Verification items for the finished model (mm, model axes). A direction names the side the tool comes from. Give positions to 0.01 mm unless a question says otherwise; leave off trailing zeros. Write each loop counter-clockwise with the first axis right and the second up, starting at its lowest first coordinate (ties: lowest second). Pieces come first, ordered by that corner, then holes. Notation, with made-up numbers: (38.25, 6) - (47.25, 6) arc R19 ccw to (47.25, 15) - close; hole circle Ø9 at (1.5, 86.25). An arc over 180 degrees is marked (long way). Answer as a JSON object with one key per item and string values. Group by question number.
Item 1: Sectioned sample at D-D, the plane x = 10. Record the boundary of the cut face in (y, z), and give its area (3 significant figures).
Item 2: Sectioned sample at C-C, the plane z = 5. Count the separate pieces of the cut face and the enclosed holes in it, and give its area (3 significant figures).
Item 3: Sectioned sample at A-A, the plane y = 0. Record the boundary of the cut face in (x, z).
Item 4: Scan lines: line 1 along X through (y, z) = (-14.5, 3.25); line 2 along X through (y, z) = (-5, 9.5); line 3 along Y through (x, z) = (12.5, 5.75). Record each from-to range of solid material in increasing order. Write a range as [from, to].
Item 5: Tool access check on faces 4 (the face through (-1.172, -8.923, 1.972)), 5 (the face through (10.373, 14.094, 5.754)), 6 (the face through (7, 10, 4)), 7 (the face through (0, -15, 10)). Record the directions out of +Z, -Z, +X, -X, +Y, -Y that give a thin tool (end or side, any length) a straight path to the whole face; none if there is none.
Item 6: Draft check along Y on faces 1 (the face through (-7.79, -9.84, 5.96)), 2 (the face through (9, 12, 10)), 3 (the face through (-7, 7, 14)). Enter one of: +Y half, -Y half, draft (parallel to the pull), parting line (faces both ways), or undercut.
Item 7: Go/stop test with flat-tipped pins: pin 1 (3.5 mm diameter, centred on x = 9.4, y = -12.94, fed in from +Z); pin 2 (2 mm diameter, centred on y = 2, z = 2, fed in from -X); pin 3 (5 mm diameter, centred on y = -13.5, z = 5, fed in from +X); pin 4 (6 mm diameter, centred on y = 9, z = 8, fed in from +X). Record where each tip stops, or that it passes through.
Item 8: Sectioned sample at B-B, the plane x = 0. Record the boundary of the cut face in (y, z), and give its area (3 significant figures).
Autodesk Fusion 360 part; units mm, degrees
sketch "Sketch1" plane through (0, 0, 0) normal (0, 0, 1) x (1, 0, 0)
  circle A0 centre (0, 0) radius 9
  circle A1 centre (0, 0) radius 16 construction
  line L0 (0, 0) -> (0, 16) construction
  circle A2 centre (0, 16) radius 3.5
  circle A3 centre (-15.2169, 4.9443) radius 3.5
  circle A4 centre (-9.4046, -12.9443) radius 3.5
  circle A5 centre (9.4046, -12.9443) radius 3.5
  circle A6 centre (15.2169, 4.9443) radius 3.5
  circle A7 centre (0, 0) radius 15
  circle A8 centre (0, 0) radius 21
  circle A9 centre (0, 0) radius 12 construction
  line L1 (0, 0) -> (-8.8168, 12.1353) construction
  circle A10 centre (-7.0534, 9.7082) radius 2
  circle A11 centre (-7.0534, 9.7082) radius 2.25 construction
  circle A12 centre (-11.4127, -3.7082) radius 2
  circle A13 centre (0, -12) radius 2
  circle A14 centre (11.4127, -3.7082) radius 2
  circle A15 centre (7.0534, 9.7082) radius 2
  line L2 (0, 0) -> (-15.2169, 4.9443) construction
  circle A16 centre (0, 16) radius 2.25
  circle A17 centre (-15.2169, 4.9443) radius 2.25
  circle A18 centre (-9.4046, -12.9443) radius 2.25
  circle A19 centre (9.4046, -12.9443) radius 2.25
  circle A20 centre (15.2169, 4.9443) radius 2.25
  circle A21 centre (0, 0) radius 8.5
  dimension "d1" = 18
  dimension "d3" = 7
  dimension "d5" = 360
  dimension "d6" = 30
  dimension "d7" = 42
  dimension "d8" = 4
  dimension "d9" = 4.5
  dimension "d10" = 24
  dimension "d12" = 360
  dimension "d13" = 36
  dimension "d14" = 72
  dimension "d17" = 4.5
  dimension "d19" = 360
  dimension "d26" = 17
  dimension "d31" = 32
extrude "Extrude1" add sketch "Sketch1" along normal blind 6 contours A2 A3 A4 A5 A6 A7 | A8
extrude "Extrude6" add sketch "Sketch1" along normal blind 14 contours A2 A3 A4 A5 A6 A7
extrude "Extrude7" add sketch "Sketch1" along normal blind 1 contours A2 A7 A16 | A2 A7 A16 | A3 A7 A17 | A3 A7 A17 | A6 A7 A20 | A6 A7 A20 | A4 A7 A18 | A4 A7 A18 | A5 A7 A19 | A5 A7 A19
extrude "Extrude4" add sketch "Sketch1" along normal blind 14 contours A0
extrude "Extrude5" cut sketch "Sketch1" along normal blind 4 contours A0
sketch "Sketch2" plane through (0, 0, 6) normal (0, 0, 1) x (-1, 0, 0)
  circle A0 centre (0, 0) radius 21
  arc A1 (-12.9338, -7.5971) -> (-3.2285, -14.6484) centre (0, 0) ccw
  arc A2 (-14.9292, -1.4561) -> (-12.9338, -7.5971) centre (-15.2169, -4.9443) ccw
  arc A3 (-11.2221, 9.9532) -> (-14.9292, -1.4561) centre (0, 0) ccw
  arc A4 (-5.9982, 13.7485) -> (-11.2221, 9.9532) centre (-9.4046, 12.9443) ccw
  arc A5 (5.9982, 13.7485) -> (-5.9982, 13.7485) centre (0, 0) ccw
  arc A6 (11.2221, 9.9532) -> (5.9982, 13.7485) centre (9.4046, 12.9443) ccw
  arc A7 (14.9292, -1.4561) -> (11.2221, 9.9532) centre (0, 0) ccw
  arc A8 (12.9338, -7.5971) -> (14.9292, -1.4561) centre (15.2169, -4.9443) ccw
  arc A9 (3.2285, -14.6484) -> (12.9338, -7.5971) centre (0, 0) ccw
  arc A10 (-3.2285, -14.6484) -> (3.2285, -14.6484) centre (0, -16) ccw
  circle A11 centre (0, 0) radius 17.5
  dimension "d36" = 35
extrude "Extrude8" cut sketch "Sketch2" against normal blind 0.5
sketch "Sketch3" plane through (0, 0, 0) normal (0, 0, -1) x (1, 0, 0)
  circle A0 centre (0, 0) radius 9
  circle A1 centre (-9.4046, 12.9443) radius 2.25
  circle A2 centre (-15.2169, -4.9443) radius 2.25
  circle A3 centre (9.4046, 12.9443) radius 2.25
  circle A4 centre (0, -16) radius 2.25
  circle A5 centre (15.2169, -4.9443) radius 2.25
  circle A6 centre (-7.0534, -9.7082) radius 2
  circle A7 centre (11.4127, 3.7082) radius 2
  circle A8 centre (0, 12) radius 2
  circle A9 centre (7.0534, -9.7082) radius 2
  circle A10 centre (-11.4127, 3.7082) radius 2
  circle A11 centre (0, 0) radius 21
extrude "Extrude9" add sketch "Sketch3" against normal blind 4 contours A6 | A7 | A8 | A9 | A10
equation "d10 = ( d6 - d1 ) / 2 + d1"
equation "d13 = d14 / 2"
Geometry check:
{
 "1": {"outline": "(-18.47, 0) - (-15.11, 0) - (-15.11, 1) - (-16.39, 1) - (-16.39, 5.5) - (-18.47, 5.5) - close; (-10.77, 0) - (18.47, 0) - (18.47, 5.5) - (14.36, 5.5) - (14.36, 6) - (11.18, 6) - (11.18, 14) - (-2.29, 14) - (-2.29, 4) - (-5.12, 4) - (-5.12, 14) - (-9.5, 14) - (-9.5, 1) - (-10.77, 1) - close", "area": "317 mm^2"},
 "2": {"separate pieces": "1", "enclosed holes": "11", "area": "903 mm^2"},
 "3": {"outline": "(-21, 0) - (-9, 0) - (-9, 4) - (-8.5, 4) - (-8.5, 14) - (-15, 14) - (-15, 6) - (-17.5, 6) - (-17.5, 5.5) - (-21, 5.5) - close; (8.5, 4) - (9, 4) - (9, 0) - (21, 0) - (21, 5.5) - (17.5, 5.5) - (17.5, 6) - (15, 6) - (15, 14) - (8.5, 14) - close"},
 "4": {"line 1": "[-15.19, -12.54], [-6.27, 6.27], [12.54, 15.19]", "line 2": "[-14.14, -12.94], [-9.89, -6.87], [6.87, 9.89], [12.94, 14.14]", "line 3": "[-11.31, -5.39], [-2.03, 2.74], [7.15, 12.25]"},
 "5": {"face 4": "-Z", "face 5": "+Z, +X, +Y", "face 6": "+Z", "face 7": "+Z, -Y"},
 "6": {"face 1": "undercut", "face 2": "+Y half", "face 3": "draft"},
 "7": {"pin 1": "through", "pin 2": "x = -20.98", "pin 3": "x = 17.89", "pin 4": "x = 19.67"},
 "8": {"outline": "(-21, 0) - (-9, 0) - (-9, 4) - (-8.5, 4) - (-8.5, 14) - (-10, 14) - (-10, 4) - (-14, 4) - (-14, 14) - (-15, 14) - (-15, 6) - (-17.5, 6) - (-17.5, 5.5) - (-21, 5.5) - close; (8.5, 4) - (9, 4) - (9, 0) - (13.75, 0) - (13.75, 1) - (12.5, 1) - (12.5, 14) - (8.5, 14) - close; (18.25, 0) - (21, 0) - (21, 5.5) - (19.5, 5.5) - (19.5, 1) - (18.25, 1) - close", "area": "148 mm^2"}
}
